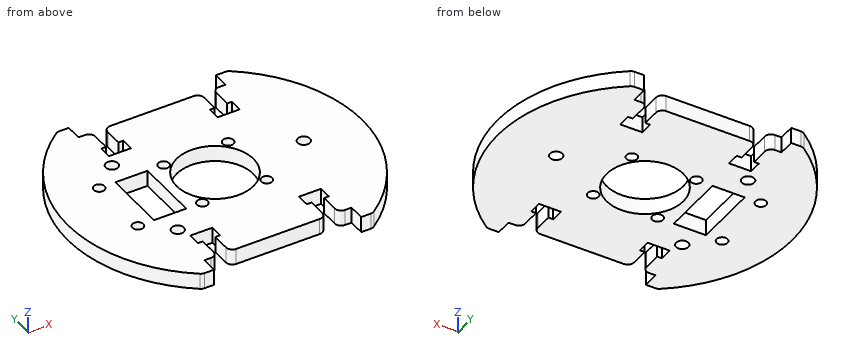
```python
from build123d import *

# Parameters (mm, degrees)
ESQUISSE1_R         = 1.925
BOSS_EXTRU_1_DEPTH  = 5
SKETCH_1_W          = 8.010899758
SKETCH_1_H          = 5.2
SKETCH_1_W_2        = 7.665468451
EXTRUDE_1_DEPTH     = 5
SKETCH_2_W          = 8.485253828
SKETCH_2_H          = 20
EXTRUDE_2_DEPTH     = 5
SKETCH_3_R          = 1.6
CUT_EXTRUDE_1_DEPTH = 5
EXTRUDE_3_DEPTH     = 5
SKETCH_6_R          = 12
SKETCH_6_W          = 10.075
SKETCH_6_H          = 20
CUT_EXTRUDE_2_DEPTH = 5
SKETCH_7_R          = 1.7
SKETCH_7_R_2        = 11
CUT_EXTRUDE_3_DEPTH = 5


with BuildPart() as part:
    # Esquisse1 → Boss.-Extru.1 (new body)
    with BuildSketch(Plane.XY):
        with BuildLine():
            Line((13.05, 32.5), (-13.05, 32.5))
            ThreePointArc((-13.05, 32.5), (-14.464213562, 31.914213562), (-15.05, 30.5))
            Line((-15.05, 30.5), (-15.05, 25))
            Line((-15.05, 25), (-13.55, 25))
            Line((-13.55, 25), (-13.55, 21))
            Line((-13.55, 21), (-20.45, 21))
            Line((-20.45, 21), (-20.45, 25))
            Line((-20.45, 25), (-18.95, 25))
            Line((-18.95, 25), (-18.95, 30.5))
            ThreePointArc((-18.95, 30.5), (-19.535786438, 31.914213562), (-20.95, 32.5))
            Line((-20.95, 32.5), (-23, 32.5))
            Line((-23, 32.5), (-23, 37.5))
            Line((-23, 37.5), (-25.999999067, 37.497633905))
            ThreePointArc((-25.999999067, 37.497633905), (-26.620839292, 37.398317642), (-27.180168114, 37.111163374))
            ThreePointArc((-27.180168114, 37.111163374), (-45.999999844, 0), (-27.180168114, -37.111163374))
            ThreePointArc((-27.180168114, -37.111163374), (-26.620839292, -37.398317642), (-25.999999067, -37.497633905))
            Line((-25.999999067, -37.497633905), (-23, -37.5))
            Line((-23, -37.5), (-23, -32.5))
            Line((-23, -32.5), (-20.95, -32.5))
            ThreePointArc((-20.95, -32.5), (-19.535786438, -31.914213562), (-18.95, -30.5))
            Line((-18.95, -30.5), (-18.95, -25))
            Line((-18.95, -25), (-20.45, -25))
            Line((-20.45, -25), (-20.45, -21))
            Line((-20.45, -21), (-13.55, -21))
            Line((-13.55, -21), (-13.55, -25))
            Line((-13.55, -25), (-15.05, -25))
            Line((-15.05, -25), (-15.05, -30.5))
            ThreePointArc((-15.05, -30.5), (-14.464213562, -31.914213562), (-13.05, -32.5))
            Line((-13.05, -32.5), (13.05, -32.5))
            ThreePointArc((13.05, -32.5), (14.464213562, -31.914213562), (15.05, -30.5))
            Line((15.05, -30.5), (15.05, -25))
            Line((15.05, -25), (13.55, -25))
            Line((13.55, -25), (13.55, -21))
            Line((13.55, -21), (20.45, -21))
            Line((20.45, -21), (20.45, -25))
            Line((20.45, -25), (18.95, -25))
            Line((18.95, -25), (18.95, -30.5))
            ThreePointArc((18.95, -30.5), (19.535786438, -31.914213562), (20.95, -32.5))
            Line((20.95, -32.5), (23, -32.5))
            Line((23, -32.5), (23, -37.5))
            Line((23, -37.5), (25.999999067, -37.497633905))
            ThreePointArc((25.999999067, -37.497633905), (26.620839292, -37.398317642), (27.180168114, -37.111163374))
            ThreePointArc((27.180168114, -37.111163374), (45.999999844, 0), (27.180168114, 37.111163374))
            ThreePointArc((27.180168114, 37.111163374), (26.620839292, 37.398317642), (25.999999067, 37.497633905))
            Line((25.999999067, 37.497633905), (23, 37.5))
            Line((23, 37.5), (23, 32.5))
            Line((23, 32.5), (20.95, 32.5))
            ThreePointArc((20.95, 32.5), (19.535786438, 31.914213562), (18.95, 30.5))
            Line((18.95, 30.5), (18.95, 25))
            Line((18.95, 25), (20.45, 25))
            Line((20.45, 25), (20.45, 21))
            Line((20.45, 21), (13.55, 21))
            Line((13.55, 21), (13.55, 25))
            Line((13.55, 25), (15.05, 25))
            Line((15.05, 25), (15.05, 30.5))
            ThreePointArc((15.05, 30.5), (14.464213562, 31.914213562), (13.05, 32.5))
        make_face()
        with Locations((27.75, 0)):
            Circle(ESQUISSE1_R, mode=Mode.SUBTRACT)
        with Locations((-21.933137835, -17)):
            Circle(ESQUISSE1_R, mode=Mode.SUBTRACT)
        with Locations((-21.933137835, 17)):
            Circle(ESQUISSE1_R, mode=Mode.SUBTRACT)
        with Locations((14.500000149, -5)):
            Circle(ESQUISSE1_R, mode=Mode.SUBTRACT)
        with Locations((14.500000149, 5)):
            Circle(ESQUISSE1_R, mode=Mode.SUBTRACT)
        with Locations((-34.499999851, -5)):
            Circle(ESQUISSE1_R, mode=Mode.SUBTRACT)
        with Locations((-34.499999851, 5)):
            Circle(ESQUISSE1_R, mode=Mode.SUBTRACT)
        with BuildLine():
            Line((10.150000149, -10), (10.150000149, -2.6))
            ThreePointArc((10.150000149, -2.6), (10.735786586, -1.185786438), (12.150000149, -0.6))
            Line((12.150000149, -0.6), (16.500000149, -0.6))
            ThreePointArc((16.500000149, -0.6), (17.100000149, 0), (16.500000149, 0.6))
            Line((16.500000149, 0.6), (12.150000149, 0.6))
            ThreePointArc((12.150000149, 0.6), (10.735786586, 1.185786438), (10.150000149, 2.6))
            Line((10.150000149, 2.6), (10.150000149, 10))
            Line((10.150000149, 10), (-30.149999851, 10))
            Line((-30.149999851, 10), (-30.149999851, 2.6))
            ThreePointArc((-30.149999851, 2.6), (-30.735786289, 1.185786438), (-32.149999851, 0.6))
            Line((-32.149999851, 0.6), (-36.499999851, 0.6))
            ThreePointArc((-36.499999851, 0.6), (-37.099999851, 0), (-36.499999851, -0.6))
            Line((-36.499999851, -0.6), (-32.149999851, -0.6))
            ThreePointArc((-32.149999851, -0.6), (-30.735786289, -1.185786438), (-30.149999851, -2.6))
            Line((-30.149999851, -2.6), (-30.149999851, -10))
            Line((-30.149999851, -10), (10.150000149, -10))
        make_face(mode=Mode.SUBTRACT)
    extrude(amount=BOSS_EXTRU_1_DEPTH)

    # 草图1 → 凸台-拉伸1 (add)
    with BuildSketch(Plane(origin=(0, 0, 0), x_dir=(-1, 0, 0), z_dir=(0, 0, -1))):
        with Locations((34.15544973, 0)):
            Rectangle(SKETCH_1_W, SKETCH_1_H)
        with Locations((-13.982734375, 0)):
            Rectangle(SKETCH_1_W_2, SKETCH_1_H)
    extrude(amount=-EXTRUDE_1_DEPTH)

    # 草图2 → 凸台-拉伸2 (add)
    with BuildSketch(Plane(origin=(0, 0, 0), x_dir=(-1, 0, 0), z_dir=(0, 0, -1))):
        Polygon((-10.150000149, 10), (-18.078472642, 10), (-18.078472642, -9.561252325), (-10.150000149, -10), align=None)
        with Locations((34.392626765, 0)):
            Rectangle(SKETCH_2_W, SKETCH_2_H)
    extrude(amount=-EXTRUDE_2_DEPTH)

    # 草图3 → 切除-拉伸1 (cut)
    with BuildSketch(Plane(origin=(0, 0, 0), x_dir=(-1, 0, 0), z_dir=(0, 0, -1))):
        with Locations((30.149999851, 10)):
            Circle(SKETCH_3_R)
        with Locations((30.149999851, -10)):
            Circle(SKETCH_3_R)
        with Locations((-10.150000149, 10)):
            Circle(SKETCH_3_R)
        with Locations((-10.150000149, -10)):
            Circle(SKETCH_3_R)
        with Locations((9.999999851, -10)):
            Circle(SKETCH_3_R)
        with Locations((9.999999851, 10)):
            Circle(SKETCH_3_R)
    extrude(amount=-CUT_EXTRUDE_1_DEPTH, mode=Mode.SUBTRACT)

    # 草图5 → 凸台-拉伸3 (add)
    with BuildSketch(Plane(origin=(0, 0, 0), x_dir=(-1, 0, 0), z_dir=(0, 0, -1))):
        with BuildLine():
            Line((30.149999851, -8.4), (30.149999851, 8.4))
            ThreePointArc((30.149999851, 8.4), (29.018629001, 8.86862915), (28.549999851, 10))
            Line((28.549999851, 10), (11.599999851, 10))
            ThreePointArc((11.599999851, 10), (9.999999851, 8.4), (8.399999851, 10))
            Line((8.399999851, 10), (-8.550000149, 10))
            ThreePointArc((-8.550000149, 10), (-9.018629299, 8.86862915), (-10.150000149, 8.4))
            Line((-10.150000149, 8.4), (-10.150000149, -8.4))
            ThreePointArc((-10.150000149, -8.4), (-9.018629299, -8.86862915), (-8.550000149, -10))
            Line((-8.550000149, -10), (8.399999851, -10))
            ThreePointArc((8.399999851, -10), (9.999999851, -8.4), (11.599999851, -10))
            Line((11.599999851, -10), (28.549999851, -10))
            ThreePointArc((28.549999851, -10), (29.018629001, -8.86862915), (30.149999851, -8.4))
        make_face()
    extrude(amount=-EXTRUDE_3_DEPTH)

    # 草图6 → 切除-拉伸2 (cut)
    with BuildSketch(Plane(origin=(0, 0, 0), x_dir=(-1, 0, 0), z_dir=(0, 0, -1))):
        Circle(SKETCH_6_R)
        with Locations((20.074999851, 0)):
            Rectangle(SKETCH_6_W, SKETCH_6_H)
    extrude(amount=-CUT_EXTRUDE_2_DEPTH, mode=Mode.SUBTRACT)

    # 草图7 → 切除-拉伸3 (cut)
    with BuildSketch(Plane(origin=(0, 0, 0), x_dir=(-1, 0, 0), z_dir=(0, 0, -1))):
        with Locations((-10.150000149, 10)):
            Circle(SKETCH_7_R)
        with Locations((9.999999851, 10)):
            Circle(SKETCH_7_R)
        with Locations((-10.150000149, -10)):
            Circle(SKETCH_7_R)
        with Locations((9.999999851, -10)):
            Circle(SKETCH_7_R)
        with Locations((30.149999851, -10)):
            Circle(SKETCH_7_R)
        with Locations((30.149999851, 10)):
            Circle(SKETCH_7_R)
        Circle(SKETCH_7_R_2)
    extrude(amount=-CUT_EXTRUDE_3_DEPTH, mode=Mode.SUBTRACT)


solid = part.part
```
Could you check a few things on this model? Use its own coordinates, in mm. Round coordinates to 2 decimals unless told otherwise and drop trailing zeros. Loops run counter-clockwise (first coordinate to the right, second up) from the corner with the lowest first, then second, coordinate; pieces in that order, holes last. Notation, with made-up numbers: (31, 61) -> (84, 61) arc R23 cw to (84, 80) -> close; hole circle Ø4 at (-33.5, -17.5). An arc over 180 degrees is marked (long way). One line per question, with ' | ' between items.
(1) If we section it at B-B on y = -31.5: List the corners of the cut face in (x, z) for me, and give its area (3 significant figures).
Model answer:
outline: (-33.52, 0) -> (-19.22, 0) -> (-19.22, 5) -> (-33.52, 5) -> close; (-14.78, 0) -> (14.78, 0) -> (14.78, 5) -> (-14.78, 5) -> close; (19.22, 0) -> (33.52, 0) -> (33.52, 5) -> (19.22, 5) -> close | area: 291 mm^2
(2) If we section it at A-A on x = 0: List the corners of the cut face in (y, z) for me.
Model answer:
outline: (-32.5, 0) -> (-12, 0) -> (-12, 5) -> (-32.5, 5) -> close; (12, 0) -> (32.5, 0) -> (32.5, 5) -> (12, 5) -> close
(3) If I drill on probe 1 along X at (y, z) = (31, 1); probe 2 along X at (y, z) = (-9, 1.1); probe 3 along Y at (x, z) = (-10, 3.2), over which ranges is the centre line in solid material (lowest first)?
Model answer:
probe 1: x = -33.99 to -19.01, -14.99 to 14.99, 19.01 to 33.99 | probe 2: x = -45.11 to -31.52, -28.78 to -25.11, -15.04 to -11.37, -8.63 to -7.94, 7.94 to 8.78, 11.52 to 45.11 | probe 3: y = -32.5 to -11.7, -8.3 to -6.63, 6.63 to 8.3, 11.7 to 32.5
(4) For pin 1 Ø19 at (x, y) = (0, 0) entering from -Z (3 decimals); pin 2 Ø1.6 at (x, z) = (-14.5, 1.5) entering from -Y; pin 3 Ø1.6 at (x, z) = (-20, 2.5) entering from -Y; pin 4 Ø1.5 at (y, z) = (-28, 3.5) entering from +X, each with a flat end and sliding along its axis, tell me the tip position at first contact or that it passes through.
Model answer:
pin 1: passes through | pin 2: stops at y = -32.39 | pin 3: stops at y = -32.49 | pin 4: stops at x = 37.06
(5) If we section it at D-D on y = 17: List the corners of the cut face in (x, z) for me.
Model answer:
outline: (-42.74, 0) -> (-23.86, 0) -> (-23.86, 5) -> (-42.74, 5) -> close; (-20.01, 0) -> (42.74, 0) -> (42.74, 5) -> (-20.01, 5) -> close
(6) If we section it at C-C on z = 2.9: Count the separate pieces of the cut face and the enclosed holes in it, and give its area (3 significant figures).
Model answer:
separate pieces: 1 | enclosed holes: 11 | area: 4,590 mm^2
